from build123d import *

# Parameters (mm, degrees)
F1_DEPTH = 1.2
F2_DEPTH = 4.8
F3_R     = 1


with BuildPart() as f1:
    # F0 (on Front) → F1 (new body)
    with BuildSketch(Plane.XZ):
        with BuildLine():
            Line((-41.4876210034, 42.7433328658), (-49.3376210034, 42.7433328658))
            ThreePointArc((-49.3376210034, 42.7433328658), (-53.1559976218, 41.1617094842), (-54.7376210034, 37.3433328658))
            Line((-54.7376210034, 37.3433328658), (-54.7376210034, 29.4933328658))
            ThreePointArc((-54.7376210034, 29.4933328658), (-53.1559976218, 25.6749562474), (-49.3376210034, 24.0933328658))
            Line((-49.3376210034, 24.0933328658), (-41.4876210034, 24.0933328658))
            ThreePointArc((-41.4876210034, 24.0933328658), (-37.669244385, 25.6749562474), (-36.0876210034, 29.4933328658))
            Line((-36.0876210034, 29.4933328658), (-36.0876210034, 37.3433328658))
            ThreePointArc((-36.0876210034, 37.3433328658), (-37.669244385, 41.1617094842), (-41.4876210034, 42.7433328658))
        make_face()
        with BuildLine():
            ThreePointArc((-49.3376210034, 24.8183328658), (-52.6433452054, 26.1876086638), (-54.0126210034, 29.4933328658))
            Line((-54.0126210034, 29.4933328658), (-54.0126210034, 37.3433328658))
            ThreePointArc((-54.0126210034, 37.3433328658), (-52.6433452054, 40.6490570679), (-49.3376210034, 42.0183328658))
            Line((-49.3376210034, 42.0183328658), (-41.4876210034, 42.0183328658))
            ThreePointArc((-41.4876210034, 42.0183328658), (-38.1818968013, 40.6490570679), (-36.8126210034, 37.3433328658))
            Line((-36.8126210034, 37.3433328658), (-36.8126210034, 29.4933328658))
            ThreePointArc((-36.8126210034, 29.4933328658), (-38.1818968013, 26.1876086638), (-41.4876210034, 24.8183328658))
            Line((-41.4876210034, 24.8183328658), (-49.3376210034, 24.8183328658))
        make_face(mode=Mode.SUBTRACT)
        with BuildLine():
            Line((-54.0126210034, 37.3433328658), (-54.0126210034, 29.4933328658))
            ThreePointArc((-54.0126210034, 29.4933328658), (-52.6433452054, 26.1876086638), (-49.3376210034, 24.8183328658))
            Line((-49.3376210034, 24.8183328658), (-41.4876210034, 24.8183328658))
            ThreePointArc((-41.4876210034, 24.8183328658), (-38.1818968013, 26.1876086638), (-36.8126210034, 29.4933328658))
            Line((-36.8126210034, 29.4933328658), (-36.8126210034, 37.3433328658))
            ThreePointArc((-36.8126210034, 37.3433328658), (-38.1818968013, 40.6490570679), (-41.4876210034, 42.0183328658))
            Line((-41.4876210034, 42.0183328658), (-49.3376210034, 42.0183328658))
            ThreePointArc((-49.3376210034, 42.0183328658), (-52.6433452054, 40.6490570679), (-54.0126210034, 37.3433328658))
        make_face()
        with BuildLine():
            Line((-52.8626210034, 29.4933328658), (-52.8626210034, 37.3433328658))
            ThreePointArc((-52.8626210034, 37.3433328658), (-51.8301724071, 39.8358842695), (-49.3376210034, 40.8683328658))
            Line((-49.3376210034, 40.8683328658), (-41.4876210034, 40.8683328658))
            ThreePointArc((-41.4876210034, 40.8683328658), (-38.9950695997, 39.8358842695), (-37.9626210034, 37.3433328658))
            Line((-37.9626210034, 37.3433328658), (-37.9626210034, 29.4933328658))
            ThreePointArc((-37.9626210034, 29.4933328658), (-38.9950695997, 27.0007814622), (-41.4876210034, 25.9683328658))
            Line((-41.4876210034, 25.9683328658), (-49.3376210034, 25.9683328658))
            ThreePointArc((-49.3376210034, 25.9683328658), (-51.8301724071, 27.0007814622), (-52.8626210034, 29.4933328658))
        make_face(mode=Mode.SUBTRACT)
        with BuildLine():
            ThreePointArc((-49.3376210034, 40.8683328658), (-51.8301724071, 39.8358842695), (-52.8626210034, 37.3433328658))
            Line((-52.8626210034, 37.3433328658), (-52.8626210034, 29.4933328658))
            ThreePointArc((-52.8626210034, 29.4933328658), (-51.8301724071, 27.0007814622), (-49.3376210034, 25.9683328658))
            Line((-49.3376210034, 25.9683328658), (-41.4876210034, 25.9683328658))
            ThreePointArc((-41.4876210034, 25.9683328658), (-38.9950695997, 27.0007814622), (-37.9626210034, 29.4933328658))
            Line((-37.9626210034, 29.4933328658), (-37.9626210034, 37.3433328658))
            ThreePointArc((-37.9626210034, 37.3433328658), (-38.9950695997, 39.8358842695), (-41.4876210034, 40.8683328658))
            Line((-41.4876210034, 40.8683328658), (-49.3376210034, 40.8683328658))
        make_face()
    extrude(amount=F1_DEPTH)

    # F0 (on Front) → F2 (join)
    with BuildSketch(Plane.XZ):
        with BuildLine():
            Line((-54.0126210034, 37.3433328658), (-54.0126210034, 29.4933328658))
            ThreePointArc((-54.0126210034, 29.4933328658), (-52.6433452054, 26.1876086638), (-49.3376210034, 24.8183328658))
            Line((-49.3376210034, 24.8183328658), (-41.4876210034, 24.8183328658))
            ThreePointArc((-41.4876210034, 24.8183328658), (-38.1818968013, 26.1876086638), (-36.8126210034, 29.4933328658))
            Line((-36.8126210034, 29.4933328658), (-36.8126210034, 37.3433328658))
            ThreePointArc((-36.8126210034, 37.3433328658), (-38.1818968013, 40.6490570679), (-41.4876210034, 42.0183328658))
            Line((-41.4876210034, 42.0183328658), (-49.3376210034, 42.0183328658))
            ThreePointArc((-49.3376210034, 42.0183328658), (-52.6433452054, 40.6490570679), (-54.0126210034, 37.3433328658))
        make_face()
        with BuildLine():
            Line((-52.8626210034, 29.4933328658), (-52.8626210034, 37.3433328658))
            ThreePointArc((-52.8626210034, 37.3433328658), (-51.8301724071, 39.8358842695), (-49.3376210034, 40.8683328658))
            Line((-49.3376210034, 40.8683328658), (-41.4876210034, 40.8683328658))
            ThreePointArc((-41.4876210034, 40.8683328658), (-38.9950695997, 39.8358842695), (-37.9626210034, 37.3433328658))
            Line((-37.9626210034, 37.3433328658), (-37.9626210034, 29.4933328658))
            ThreePointArc((-37.9626210034, 29.4933328658), (-38.9950695997, 27.0007814622), (-41.4876210034, 25.9683328658))
            Line((-41.4876210034, 25.9683328658), (-49.3376210034, 25.9683328658))
            ThreePointArc((-49.3376210034, 25.9683328658), (-51.8301724071, 27.0007814622), (-52.8626210034, 29.4933328658))
        make_face(mode=Mode.SUBTRACT)
    extrude(amount=-F2_DEPTH)

    # F3
    f3_edges = [f1.edges().sort_by_distance(p)[0] for p in [
        (-37.669244, -1.2, 41.161709),
    ]]
    fillet(f3_edges, radius=F3_R)


solid = f1.part
For this review, take the finished solid that the model builds, in its own axes (mm). A direction names the side the tool comes from. Coordinates: 2 decimals unless noted, no trailing zeros. Order: outer loops, then holes, each group sorted by start corner. A loop starts at its lowest first (then second) coordinate and runs counter-clockwise, first axis right, second up. Notation, with made-up numbers: (64.5, -16) -> (110.5, -16) arc R24 cw to (110.5, 12) -> close; hole circle Ø3 at (-28.75, 24). An arc over 180 degrees is marked (long way). Return JSON: item names as keys, results as strings.
1. We need section B-B on z = 30.25. Write out the cut boundary in (x, y), and give its area (3 significant figures).
Answer block:
{"outline": "(-54.74, -0.2) arc R1 ccw to (-53.74, -1.2) -> (-37.09, -1.2) arc R1 ccw to (-36.09, -0.2) -> (-36.09, 0) -> (-36.81, 0) -> (-36.81, 4.8) -> (-37.96, 4.8) -> (-37.96, 0) -> (-52.86, 0) -> (-52.86, 4.8) -> (-54.01, 4.8) -> (-54.01, 0) -> (-54.74, 0) -> close", "area": "33.0 mm²"}
2. We need section D-D on y = -0.5. Write out the cut boundary in (x, z).
Answer block:
{"outline": "(-54.69, 29.49) arc R5.35 ccw to (-49.34, 24.14) -> (-41.49, 24.14) arc R5.35 ccw to (-36.13, 29.49) -> (-36.13, 37.34) arc R5.35 ccw to (-41.49, 42.7) -> (-49.34, 42.7) arc R5.35 ccw to (-54.69, 37.34) -> close"}
3. For pin 1 Ø2.5 at (y, z) = (2.5, 35) entering from +X; pin 2 Ø1.4 at (x, y) = (-47, 1.5) entering from +Z; pin 3 Ø7.5 at (x, z) = (-46, 30) entering from +Y, all flat-tipped, find the tip position at first contact; note any pin that passes through.
Answer block:
{"pin 1": "x = -36.81", "pin 2": "z = 42.02", "pin 3": "y = 0"}
4. We need section A-A on y = 4. Write out the cut boundary in (x, z) (3 decimals), and give its area (3 significant figures).
Answer block:
{"outline": "(-54.013, 29.493) arc R4.675 ccw to (-49.338, 24.818) -> (-41.488, 24.818) arc R4.675 ccw to (-36.813, 29.493) -> (-36.813, 37.343) arc R4.675 ccw to (-41.488, 42.018) -> (-49.338, 42.018) arc R4.675 ccw to (-54.013, 37.343) -> close; hole (-52.863, 29.493) arc R3.525 ccw to (-49.338, 25.968) -> (-41.488, 25.968) arc R3.525 ccw to (-37.963, 29.493) -> (-37.963, 37.343) arc R3.525 ccw to (-41.488, 40.868) -> (-49.338, 40.868) arc R3.525 ccw to (-52.863, 37.343) -> close", "area": "65.7 mm²"}
5. We need section C-C on x = -42. Write out the cut boundary in (y, z).
Answer block:
{"outline": "(-1.2, 25.09) arc R1 ccw to (-0.2, 24.09) -> (0, 24.09) -> (0, 24.82) -> (4.8, 24.82) -> (4.8, 25.97) -> (0, 25.97) -> (0, 40.87) -> (4.8, 40.87) -> (4.8, 42.02) -> (0, 42.02) -> (0, 42.74) -> (-0.2, 42.74) arc R1 ccw to (-1.2, 41.74) -> close"}
6. Machinability: for faces 4 (the flat face through (-45, 2, 40.868)), 5 (the flat face through (-45, 2, 24.818)), 6 (the cylindrical face through (-45.36, -0.9, 24.38)), 7 (the cylindrical face through (-38.22, 2.37, 26.15)), which of the approach directions +Z, -Z, +X, -X, +Y, -Y give a long, thin tool a straight path to every point of the face, cutting with its end or side? Answer none if there is none.
Answer block:
{"face 4": "+Y", "face 5": "-Z, +X, -X, +Y", "face 6": "-Z, +X, -X, -Y", "face 7": "-Z, +X, +Y"}
7. The part is to be moulded in two halves that separate along X. For faces 1 (the cylindrical face through (-52.679, 2.366, 26.224)), 2 (the flat face through (-36.813, 2, 33)), 3 (the cylindrical face through (-38.968, 2.366, 27.028)), say which applies: +X half, -X half, draft (parallel to the pull), parting line (faces both ways), or undercut.
Answer block:
{"face 1": "-X half", "face 2": "+X half", "face 3": "undercut"}
8. For line 1 (Z direction, x = -47, y = 2.5); line 2 (X direction, y = 1.75, z = 31); line 3 (Y direction, x = -45, z = 35.5), list the stretches that pass through material, from the lowest coordinate up. Write a range as from..to.
Answer block:
{"line 1": "24.82..25.97, 40.87..42.02", "line 2": "-54.01..-52.86, -37.96..-36.81", "line 3": "-1.2..0"}
